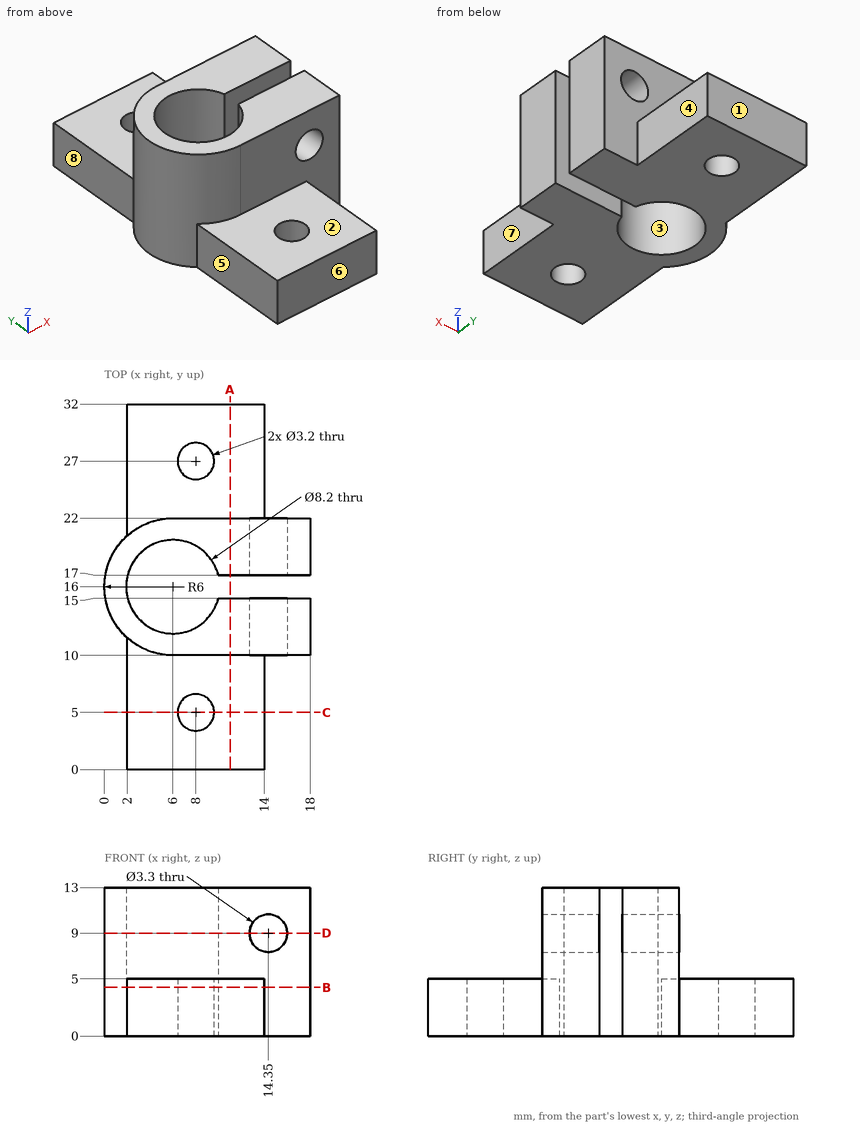
Job drawing, mm, ordinate dimensions from the low corner. One solid piece. A direction names the side the tool comes from. Give positions to 0.01 mm unless a question says otherwise; leave off trailing zeros. Order: outer loops, then holes, each group sorted by start corner. A loop starts at its lowest first (then second) coordinate and runs counter-clockwise, first axis right, second up. Notation, with made-up numbers: (-15, 34) - (-1, 34) arc R22 ccw to (-1, 60) - close; hole circle Ø8 at (18.5, 63.5). An arc over 180 degrees is marked (long way). Return JSON: item names as keys, results as strings.
1) Cut at C-C, the plane y = 5. Give the cut face in (x, z).
Geometry says:
{"outline": "(2, 0) - (6.4, 0) - (6.4, 5) - (2, 5) - close; (9.6, 0) - (14, 0) - (14, 5) - (9.6, 5) - close"}
2) Cut at B-B, the plane z = 4.25. Give the cut face in (x, y), plus the area to 3 significant figures.
Geometry says:
{"outline": "(2, 0) - (14, 0) - (14, 10) - (18, 10) - (18, 15) - (9.98, 15) arc R4.1 cw (long way) to (9.98, 17) - (18, 17) - (18, 22) - (14, 22) - (14, 32) - (2, 32) - (2, 20.47) arc R6 ccw to (2, 11.53) - close; hole circle Ø3.2 at (8, 5); hole circle Ø3.2 at (8, 27)", "area": "360 mm²"}
3) Pull direction Y, two halves, no side cores. Call the marked faces 1, 2 and 3: pulls with the +Y half, pulls with the -Y half, needs draft (parallel to the pull), parting line crosses it, or undercut.
Geometry says:
{"face 1": "pulls with the +Y half", "face 2": "needs draft", "face 3": "undercut"}
4) Probe line 1 (Y direction, x = 16.75, z = 9.25); line 2 (Y direction, x = 8.25, z = 2); line 3 (Y direction, x = 8, z = 2.2). List the from-to ranges inside material, lowest first. Write a range as from..to.
Geometry says:
{"line 1": "10..15, 17..22", "line 2": "0..3.42, 6.58..12.57, 19.43..25.42, 28.58..32", "line 3": "0..3.4, 6.6..12.42, 19.58..25.4, 28.6..32"}
5) Flat gauge pins, fed straight in: P1, Ø4, axis at y = 26, z = 1.5, coming from the +X side; P2, Ø1.5, axis at x = 10.5, z = 9.5, coming from the -Y side; P3, Ø2, axis at x = 7, z = 4, coming from the -Y side; P4, Ø5.5, axis at y = 23.5, z = 3.5, coming from the -X side. Where does each tip first touch, or does it go through?
Geometry says:
{"P1": "x = 14", "P2": "y = 10", "P3": "y = 0", "P4": "x = 2"}
6) 3-axis set-ups, long thin cutter, end or side, ignore diameter. For the marked faces 4, 5, 6, 7 and 8: which of +Z, -Z, +X, -X, +Y, -Y reach the whole face in a straight line?
Geometry says:
{"face 4": "+Z, -Z, +X, +Y", "face 5": "+Z, -Z, -X, -Y", "face 6": "+Z, -Z, +X, -X, -Y", "face 7": "+Z, -Z, +X, -Y", "face 8": "+Z, -Z, -X, +Y"}
7) Cut at A-A, the plane x = 11. Give the cut face in (y, z), plus the area to 3 significant figures.
Geometry says:
{"outline": "(0, 0) - (15, 0) - (15, 13) - (10, 13) - (10, 5) - (0, 5) - close; (17, 0) - (32, 0) - (32, 5) - (22, 5) - (22, 13) - (17, 13) - close", "area": "230 mm²"}
8) Cut at D-D, the plane z = 9. Give the cut face in (x, y), plus the area to 3 significant figures.
Geometry says:
{"outline": "(6, 10) - (12.7, 10) - (12.7, 15) - (9.98, 15) arc R4.1 cw (long way) to (9.98, 17) - (12.7, 17) - (12.7, 22) - (6, 22) arc R6 ccw to start; (16, 10) - (18, 10) - (18, 15) - (16, 15) - close; (16, 17) - (18, 17) - (18, 22) - (16, 22) - close", "area": "98.9 mm²"}
